Read the model definition and answer for the solid it produces. Units are mm, in the model's axes. A direction names the side the tool comes from. Coordinates: 2 decimals unless noted, no trailing zeros. Order: outer loops, then holes, each group sorted by start corner. A loop starts at its lowest first (then second) coordinate and runs counter-clockwise, first axis right, second up. Notation, with made-up numbers: (19, -40) - (28, -40) arc R25 ccw to (28, -14) - close; hole circle Ø7 at (79.5, 63). An arc over 180 degrees is marked (long way). Use one line per item in the form item = value. Start each with the question number.
Autodesk Inventor part; units mm, degrees
ref_plane "YZ Plane" through (0, 0, 0) normal (1, 0, 0) x (0, 1, 0)
ref_plane "XZ Plane" through (0, 0, 0) normal (0, 1, 0) x (-1, 0, 0)
ref_plane "XY Plane" through (0, 0, 0) normal (0, 0, 1) x (1, 0, 0)
sketch "Boceto1" plane through (0, 0, 0) normal (0, 1, 0) x (-1, 0, 0)
  circle A0 centre (0, 0) radius 4.5
  dimension "d0" = 9
extrude "Extrusión1" add sketch "Boceto1" along normal blind 1
fillet "Empalme1" radius 0.5 1 edges at (4.5, 1, 0)
sketch "Boceto2" plane through (0, 0, 0) normal (0, -1, 0) x (1, 0, 0)
  circle A0 centre (0, 0) radius 3.9
  dimension "d4" = 7.8
extrude "Extrusión2" add sketch "Boceto2" along normal blind 2
fillet "Empalme2" radius 0.5 1 edges at (-3.9, -2, 0)
properties part number "sensor_2"
Q1. A cutting plane is placed at C-C (y = 0.15). Give the vertices of the cut face in (x, z).
Q2. Which of the six approach directions +Z, -Z, +X, -X, +Y, -Y give full straight-line access (tool end or side, diameter ignored) to faces 1 (the cylindrical face through (0.59, 0.25, -4.46)), 2 (the cylindrical face through (-2.87, -0.74, -2.64))?
Q3. A cutting plane is placed at A-A (x = 0). Give the vertices of the cut face in (y, z).
Q4. Given P1, Ø1.5, axis at y = 0.5, z = -1.5, coming from the +X side; P2, Ø5, axis at x = 2.5, z = -2.5, coming from the -Y side, each flat-ended and moving along its own axis, determine where each tip first touches the part or whether it passes through.
Q5. Consider probe 1 along Y at (x, z) = (-0.5, -4); probe 2 along X at (y, z) = (0.45, 2.25); probe 3 along X at (y, z) = (0.05, -1). Determine where each line is inside the solid, lowest interval first.
Q6. A cutting plane is placed at B-B (z = 0). Give the vertices of the cut face in (x, y).
Result sheet:
q1.outline = circle Ø9 at (0, 0)
q2.face_1 = +Y, -Y
q2.face_2 = -Y
q3.outline = (-2, -3.4) arc R0.5 ccw to (-1.5, -3.9) - (0, -3.9) - (0, -4.5) - (0.5, -4.5) arc R0.5 ccw to (1, -4) - (1, 4) arc R0.5 ccw to (0.5, 4.5) - (0, 4.5) - (0, 3.9) - (-1.5, 3.9) arc R0.5 ccw to (-2, 3.4) - close
q4.P1 = 4.44
q4.P2 = -2
q5.probe_1 = 0 to 1
q5.probe_2 = -3.9 to 3.9
q5.probe_3 = -4.39 to 4.39
q6.outline = (-4.5, 0) - (-3.9, 0) - (-3.9, -1.5) arc R0.5 ccw to (-3.4, -2) - (3.4, -2) arc R0.5 ccw to (3.9, -1.5) - (3.9, 0) - (4.5, 0) - (4.5, 0.5) arc R0.5 ccw to (4, 1) - (-4, 1) arc R0.5 ccw to (-4.5, 0.5) - close
